Answer from the drawing. Dimensions are ordinates in mm from the lowest x, y and z of the part. A direction names the side the tool comes from. Give positions to 0.01 mm unless a question says otherwise; leave off trailing zeros. Order: outer loops, then holes, each group sorted by start corner. A loop starts at its lowest first (then second) coordinate and runs counter-clockwise, first axis right, second up. Notation, with made-up numbers: (82.5, 31.25) - (96.5, 31.25) arc R28 cw to (96.5, 59.25) - close; hole circle Ø5 at (58, 34.25). An arc over 180 degrees is marked (long way). Answer in a Markdown table with one row per item. Add a question column.
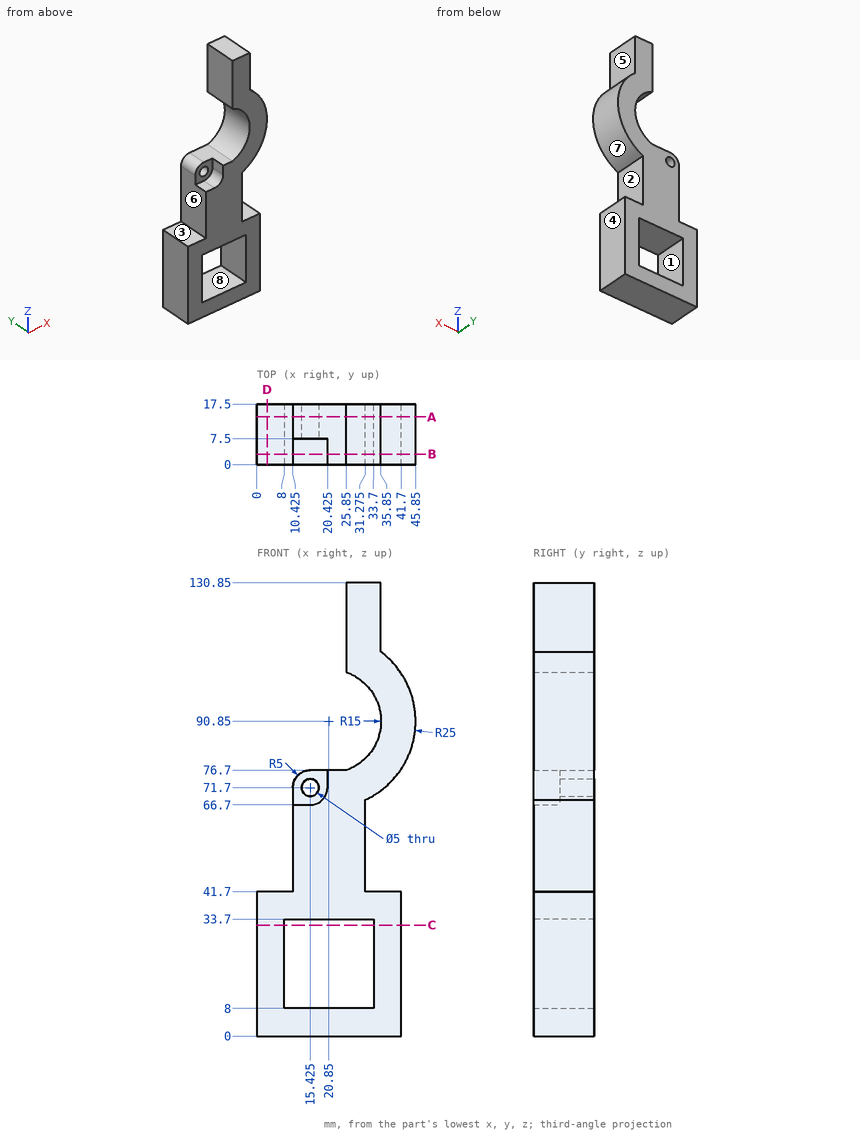
(1) Find section A-A, the plane y = 13.75. Write down the section's boundary in (x, z) (3 decimals).
(2) Each of these flat-tipped pins is pushed along its axis until it touches: P1, Ø5, axis at y = 11, z = 59, coming from the +X side (3 decimals); P2, Ø5, axis at y = 9, z = 116, coming from the -X side; P3, Ø5, axis at y = 10.5, z = 18.5, coming from the +X side; P4, Ø8, axis at y = 7, z = 15.5, coming from the -X side. Where does it stop, or does it pass through?
(3) Find section B-B, the plane y = 3. Write down the section's boundary in (x, z) (3 decimals), plus the area to 3 significant figures.
(4) Find section D-D, the plane x = 3. Write down the section's boundary in (y, z).
(5) For the marked faces 1, 2, 3, 4 and 5, determine the directions among +Z, -Z, +X, -X, +Y, -Y from which every point of the face is accessible in a straight line to the end or side of a thin tool.
(6) The mould has two halves that part along X. Classify the marked faces 6, 7 and 8: +X half, -X half, draft (parallel to the pull), parting line (faces both ways), or undercut.
(7) Straight lines are drawn through the part: line 1 (Z direction, x = 23, y = 15.75); line 2 (Z direction, x = 26.5, y = 4.5); line 3 (Z direction, x = 31.5, y = 8.25). For each, find the intervals that lie inside material, in ascending order.
(8) Find section C-C, the plane z = 32. Write down the section's boundary in (x, y), plus the area to 3 significant figures.
Answer key:
| question | item | result |
|---|---|---|
| 1 | outline | (0, 0) - (41.7, 0) - (41.7, 41.7) - (31.275, 41.7) - (31.275, 68.127) arc R25 ccw to (35.85, 110.85) - (35.85, 130.85) - (25.85, 130.85) - (25.85, 104.992) arc R15 cw to (25.828, 76.7) - (15.425, 76.7) arc R5 ccw to (10.425, 71.7) - (10.425, 41.7) - (0, 41.7) - close; hole (8, 8) - (33.7, 8) - (33.7, 33.7) - (8, 33.7) - close; hole circle Ø5 at (15.425, 71.7) |
| 2 | P1 | x = 31.275 |
| 2 | P2 | x = 25.85 |
| 2 | P3 | x = 41.7 |
| 2 | P4 | x = 0 |
| 3 | outline | (0, 0) - (41.7, 0) - (41.7, 41.7) - (31.275, 41.7) - (31.275, 68.127) arc R25 ccw to (35.85, 110.85) - (35.85, 130.85) - (25.85, 130.85) - (25.85, 104.992) arc R15 cw to (25.828, 76.7) - (20.425, 76.7) - (20.425, 71.7) arc R5 cw to (15.425, 66.7) - (10.425, 66.7) - (10.425, 41.7) - (0, 41.7) - close; hole (8, 8) - (33.7, 8) - (33.7, 33.7) - (8, 33.7) - close |
| 3 | area | 2,360 mm² |
| 4 | outline | (0, 0) - (17.5, 0) - (17.5, 41.7) - (0, 41.7) - close |
| 5 | face 1 | +Y, -Y |
| 5 | face 2 | +X, +Y, -Y |
| 5 | face 3 | +Z, -X, +Y, -Y |
| 5 | face 4 | -Z, +X, +Y, -Y |
| 5 | face 5 | +Z, +X, +Y, -Y |
| 6 | face 6 | -X half |
| 6 | face 7 | +X half |
| 6 | face 8 | undercut |
| 7 | line 1 | 0 to 8, 33.7 to 76.7 |
| 7 | line 2 | 0 to 8, 33.7 to 76.95, 104.75 to 130.85 |
| 7 | line 3 | 0 to 8, 33.7 to 41.7, 68.23 to 80.29, 101.41 to 130.85 |
| 8 | outline | (0, 0) - (8, 0) - (8, 17.5) - (0, 17.5) - close; (33.7, 0) - (41.7, 0) - (41.7, 17.5) - (33.7, 17.5) - close |
| 8 | area | 280 mm² |
